from build123d import *

# Parameters (mm, degrees)
F1_DEPTH = 5
F3_D     = 5.1
F4_R     = 2.1
F5_DEPTH = 25


with BuildPart() as f1:
    # F0 (on Top) → F1 (new body)
    with BuildSketch(Plane.XY):
        with BuildLine():
            Line((84.6812899327, 58.5268347502), (-92.3187100673, 58.5268347502))
            Line((-92.3187100673, 58.5268347502), (-92.3187100673, 8.5268347502))
            Line((-92.3187100673, 8.5268347502), (-92.3187100673, -51.4731652498))
            Line((-92.3187100673, -51.4731652498), (-54.3187100673, -51.4731652498))
            Line((-54.3187100673, -51.4731652498), (-54.3187100673, -1.4731652498))
            ThreePointArc((-54.3187100673, -1.4731652498), (-51.3897778791, 5.597902562), (-44.3187100673, 8.5268347502))
            Line((-44.3187100673, 8.5268347502), (36.6812899327, 8.5268347502))
            ThreePointArc((36.6812899327, 8.5268347502), (43.7523577446, 5.597902562), (46.6812899327, -1.4731652498))
            Line((46.6812899327, -1.4731652498), (46.6812899327, -51.4731652498))
            Line((46.6812899327, -51.4731652498), (84.6812899327, -51.4731652498))
            Line((84.6812899327, -51.4731652498), (84.6812899327, 8.5268347502))
            Line((84.6812899327, 8.5268347502), (84.6812899327, 58.5268347502))
        make_face()
    extrude(amount=F1_DEPTH)

    # F3 (through all)
    with Locations(Plane.XY.offset(5)):
        with Locations((-10.8187100673, 27.5268347502), (-3.8187100673, 48.5268347502), (3.1812899327, 27.5268347502), (-3.8187100673, 15.2268347502)):
            Hole(F3_D / 2)

    # F4 (on face) → F5 (cut)
    with BuildSketch(Plane.XY.offset(5)):
        with Locations((-63.3187100673, -6.4731652498)):
            Circle(F4_R)
        with Locations((55.6812899327, -14.4731652498)):
            Circle(F4_R)
        with Locations((-83.3187100673, -14.4731652498)):
            Circle(F4_R)
        with Locations((-73.3187100673, -43.9731652498)):
            Circle(F4_R)
        with Locations((75.6812899327, -6.4731652498)):
            Circle(F4_R)
        with Locations((65.6812899327, -43.9731652498)):
            Circle(F4_R)
    extrude(amount=-F5_DEPTH, mode=Mode.SUBTRACT)


solid = f1.part
Read the model definition and answer for the solid it produces. Units are mm, in the model's axes. A direction names the side the tool comes from. Round coordinates to 2 decimals unless told otherwise and drop trailing zeros. Order: outer loops, then holes, each group sorted by start corner. A loop starts at its lowest first (then second) coordinate and runs counter-clockwise, first axis right, second up.
1) The mould has two halves that part along Y. Classify faces 1 (the face through (-3, 58.527, 2)), 2 (the face through (57.62, -15.28, 2.54)), 3 (the face through (-54.319, -27, 2)): released by +Y, released by -Y, zero draft, split by the parting line, or undercut.
2) For faces 4 (the face through (-51.467, 5.52, 2.465)), 5 (the face through (65.41, -41.89, 2.54)), determine the directions among +Z, -Z, +X, -X, +Y, -Y from which every point of the face is accessible in a straight line to the end or side of a thin tool.
3) The part is cut by section D-D on x = 23.5. Write down the section's boundary in (y, z).
4) Straight lines are drawn through the part: L1, parallel to X at y = -14.5, z = 4.1; L2, parallel to Y at x = -83, z = 0.5; L3, parallel to X at y = -28.5, z = 2.9. For each, find the intervals that lie inside material, in ascending order.
5) The part is cut by section C-C on z = 1.2. Give the number of separate pieces and of enclosed holes in the cut face, plus the area to 3 significant figures.
6) The part is cut by section B-B on x = 3. Write down the section's boundary in (y, z).
7) The part is cut by section A-A on y = -20.5. Write down the section's boundary in (x, z).
Resolved:
1. face 1: released by +Y
1. face 2: undercut
1. face 3: zero draft
2. face 4: +Z, -Z, -Y
2. face 5: +Z, -Z
3. outline: (8.53, 0) - (58.53, 0) - (58.53, 5) - (8.53, 5) - close
4. L1: x = -92.32 to -85.42, -81.22 to -54.32, 46.68 to 53.58, 57.78 to 84.68
4. L2: y = -51.47 to -16.55, -12.4 to 58.53
4. L3: x = -92.32 to -54.32, 46.68 to 84.68
5. separate pieces: 1
5. enclosed holes: 10
5. area: 13,300 mm2
6. outline: (8.53, 0) - (24.98, 0) - (24.98, 5) - (8.53, 5) - close; (30.07, 0) - (58.53, 0) - (58.53, 5) - (30.07, 5) - close
7. outline: (-92.32, 0) - (-54.32, 0) - (-54.32, 5) - (-92.32, 5) - close; (46.68, 0) - (84.68, 0) - (84.68, 5) - (46.68, 5) - close
